Check sheet for the modelled part. Datum: model origin and axes. Units: mm. Face numbers are marked on the shaded views. A direction names the side the tool comes from. Coordinates: 2 decimals unless noted, no trailing zeros. Loops run counter-clockwise (first coordinate to the right, second up) from the corner with the lowest first, then second, coordinate; pieces in that order, holes last. Notation, with made-up numbers: M 27,-2.75 L 41,-2.75 A24 cw 41,15.25 Z; hole C -35,89.5 d1. An arc over 180 degrees is marked long. Write each question's results on one line, items separated by ' | '. Start each with the question number.
Autodesk Inventor part; units mm, degrees
ref_plane "Work Plane1" through (-69.6848, 0, 13.4826) normal (-0.0507, 0, 0.9987) x (0.9987, 0, 0.0507)
ref_plane "YZ Plane" through (0, 0, 0) normal (1, 0, 0) x (0, 1, 0)
ref_plane "XZ Plane" through (0, 0, 0) normal (0, 1, 0) x (-1, 0, 0)
sketch "Sketch1" plane through (0, 0, 0) normal (0, 1, 0) x (-1, 0, 0)
  circle A0 centre (0, 0) radius 19.5
  line L0 (0, 0) -> (69, 0) construction
  circle A1 centre (69, 0) radius 16
  line L1 (69.8116, -15.9794) -> (0.9891, -19.4749)
  line L2 (69.8116, 15.9794) -> (0.9891, 19.4749)
  point P0 (0.9891, 19.4749)
  dimension "d0" = 39
  dimension "d1" = 32
  dimension "d2" = 69
extrude "Extrusion1" add sketch "Sketch1" along normal blind 2.5 contours A0 L2 A1 L1 | A1
sketch "Sketch3" plane through (0, 0, 0) normal (0, 0, 1) x (1, 0, 0)
  line L0 (0, 0) -> (0, 29.1077)
  line L1 (0, 22) -> (-16.5, 22)
  line L2 (-16.5, 22) -> (-16.5, 44)
  line L3 (-16.5, 44) -> (-19.5, 44)
  line L4 (-19.5, 44) -> (-19.5, 2.5)
  line L5 (-19.5, 2.5) -> (-0.9891, 2.5)
  line L6 (-19.5, 2.5) -> (-19.5, 0)
  line L7 (-19.5, 0) -> (-16.5, 0)
  line L8 (-19.5, 0) -> (-0.9891, 0)
  line L9 (-16.5, 0) -> (-16.5, 18)
  line L10 (-16.5, 18) -> (0, 18)
  line L11 (-18, 44) -> (-18, 42)
  line L12 (-18, 42) -> (-19.5, 42)
  line L13 (-4, 18) -> (-4, 19)
  line L14 (-4, 19) -> (-11, 19)
  line L15 (-11, 19) -> (-11, 22)
  point P0 (-16.5, 2.5)
  dimension "d5" = 44
  dimension "d6" = 2
  dimension "d7" = 18
  dimension "d8" = 16.5
  dimension "d10" = 4
  dimension "d11" = 3
  dimension "d12" = 22
  dimension "d13" = 11
  dimension "d14" = 1
revolve "Revolution1" add sketch "Sketch3" angle 360 about axis through (0, 0, 0) along (0, 1, 0) contours L10 L9 L5 L4 L12 L11 L3 L2 L1 L15 L14 L13 | L9 L7 L6 L5
sketch "Sketch4" plane through (0, 2.5, 0) normal (0, 1, 0) x (1, 0, 0)
  line L0 (0, 0) -> (-85, 0)
  arc A0 (-69.8116, 15.9794) -> (-69.8116, -15.9794) centre (-69, 0) ccw
  circle A1 centre (-46.5, 0) radius 7
  circle A2 centre (-69, 0) radius 7
  dimension "d17" = 46.5
  dimension "d18" = 22.5
  dimension "d19" = 14
extrude "Extrusion2" add sketch "Sketch4" along normal blind 2.5
ref_plane "Work Plane1" through (-69.6848, 0, 13.4826) normal (-0.0507, 0, 0.9987) x (0.9987, 0, 0.0507)
sketch "Sketch6" plane through (-69.6848, 0, 13.4826) normal (-0.0507, 0, 0.9987) x (0.9987, 0, 0.0507)
  line L0 (68.9112, 0) -> (68.9112, 13.5)
  line L1 (68.9112, 13.5) -> (49.4112, 13.5)
  line L2 (49.4112, 13.5) -> (29.471, 5)
  line L3 (29.471, 5) -> (7, 5)
  line L4 (7, 5) -> (0, 2.5)
  line L5 (66.9355, 2.5) -> (-1.6211, 2.5)
  line L6 (29.471, 2.5) -> (29.471, 5)
  line L7 (7, 2.5) -> (7, 5)
  line L8 (49.4112, 2.5) -> (49.4112, 42)
  line L9 (7, 5) -> (-7, 5)
  line L10 (0, 5) -> (0, 18.3194) construction
  line L11 (66.9355, 0) -> (-1.6211, 0)
  line L12 (66.9355, 2.5) -> (68.9112, 2.5)
  dimension "d23" = 13.5
  dimension "d24" = 5
extrude "Extrusion3" add sketch "Sketch6" along normal blind 2.5
mirror "Mirror1" about plane through (0, 0, 0) normal (0, 0, 1) of "Extrusion3"
sketch "Sketch7" plane through (0, 0, 0) normal (0, 0, 1) x (1, 0, 0)
  line L0 (-17.1617, 6.6953) -> (-62, 2.52)
  line L1 (-62, 2.5) -> (-62, 5)
  line L2 (-62, 2.52) -> (-62, 2.5)
  line L3 (-10.4025, 2.5) -> (-69.6848, 2.5)
  line L4 (-17.1617, 2.5) -> (-62, 2.5)
  line L5 (-17.1617, 2.5) -> (-17.1617, 6.6953)
  line L6 (-0.9891, 0) -> (-69.8116, 0)
  line L7 (-62, 2.52) -> (-62.2148, 2.5)
  point P0 (0, 0)
  dimension "d27" = 5.32
  dimension "d28" = 2.52
extrude "Extrusion4" add sketch "Sketch7" along normal mid plane 3.5
sketch "Sketch8" plane through (-46.5, 5, 0) normal (0, 1, 0) x (1, 0, 0)
  arc A0 (-6.7777, -1.75) -> (6.7777, -1.75) centre (0, 0) ccw
  circle A1 centre (0, 0) radius 3
  arc A2 (-15.7148, 1.7207) -> (-15.7148, -1.7207) centre (-22.5, 0) ccw
  circle A3 centre (-22.5, 0) radius 3
  point P0 (46.5, 0)
  point P1 (-15.5, 0)
  dimension "d31" = 6
extrude "Extrusion5" cut sketch "Sketch8" against normal through all
sketch "Sketch9" plane through (0, 44, 0) normal (0, 1, 0) x (1, 0, 0)
  circle A0 centre (0, -16) radius 4.5
  line L0 (0, 0) -> (24.199, 0) construction
  circle A1 centre (0, 0) radius 16.5
  circle A2 centre (0, 16) radius 4.5
  point P0 (-4.4983, 15.875)
  point P1 (4.4983, 15.875)
  point P2 (-4.4983, -15.875)
  point P3 (4.4983, -15.875)
  dimension "d34" = 9
  dimension "d35" = 16
extrude "Extrusion6" add sketch "Sketch9" against normal up to surface (22 mm away) contours A1 A0 | A1 A2 picked at (-0.1776, -14.7973) picked at (-0.1776, 14.7973)
sketch "Sketch10" plane through (0, 44, 0) normal (0, 1, 0) x (1, 0, 0)
  arc A0 (4.4983, -15.875) -> (-4.4983, -15.875) centre (0, -16) ccw
  circle A1 centre (0, -16) radius 1.5
  line L0 (0, 0) -> (9.3395, 0) construction
  circle A2 centre (0, 16) radius 1.5
  dimension "d38" = 3
extrude "Extrusion7" cut sketch "Sketch10" against normal blind 4
sketch "Sketch11" plane through (0, 0, 0) normal (0, -1, 0) x (1, 0, 0)
  circle A0 centre (0, 16) radius 1.5
  circle A1 centre (0, 16) radius 2.5
  line L0 (0, 0) -> (10.318, 0)
  circle A2 centre (0, -16) radius 2.5
  dimension "d41" = 5
extrude "Extrusion8" cut sketch "Sketch11" against normal up to surface (40 mm away) contours A0 | A1 | A2
sketch "Sketch12" plane through (0, 44, 0) normal (0, 1, 0) x (1, 0, 0)
  line L0 (36.079, 0) -> (-96.4154, 0)
  line L1 (-96.4154, 0) -> (-96.4154, 28.1723)
  line L2 (-96.4154, 28.1723) -> (36.079, 28.1723)
  line L3 (36.079, 28.1723) -> (36.079, 0)
  point P0 (0, 0)
properties part number "pt1" material "Stainless Steel"
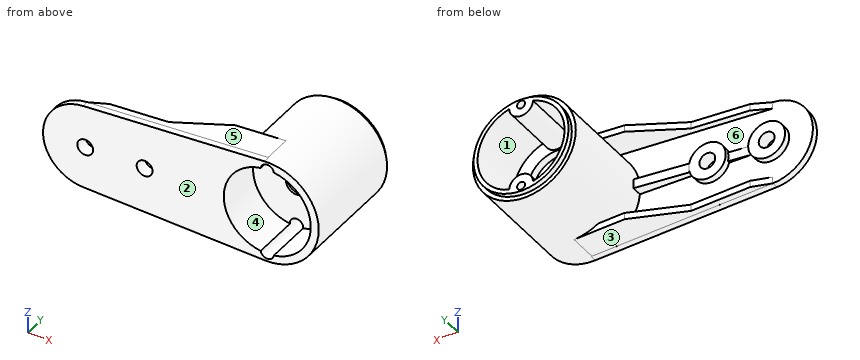
Item 1: Depth check by flat-ended pin: P1, Ø3, axis at x = -72.5, z = -15, coming from the +Y side; P2, Ø2.5, axis at x = 0, z = -16, coming from the -Y side; P3, Ø2, axis at y = 27, z = 10, coming from the -X side; P4, Ø6, axis at y = 28.5, z = 5.5, coming from the +X side. Enter the tip coordinate at first touch or a pass-through.
Item 2: Section check B-B (y = 14.5). Record the cut outline in (x, z).
Item 3: Release check for a two-part mould opening along X. For the marked faces 1, 2 and 3 record: +X half, -X half, draft (parallel to the pull), parting line (faces both ways), or undercut.
Item 4: Section check C-C (x = 0). State how many separate pieces and enclosed holes the cut face has, plus the area to 3 significant figures.
Item 5: Thickness scan on line 1 (Z direction, x = 0, y = 20); line 2 (Z direction, x = 0, y = 41.6); line 3 (Z direction, x = -69, y = 3). Record the ranges inside material, lowest first.
Item 6: Tool access check on the marked faces 4, 5 and 6. Record the directions out of +Z, -Z, +X, -X, +Y, -Y that give a thin tool (end or side, any length) a straight path to the whole face; none if there is none.
Item 7: Section check A-A (y = 33.5). Record the cut outline in (x, z) (3 decimals), plus the area to 3 significant figures.
Computed values:
1) P1: stops at y = 2.5 | P2: passes through | P3: stops at x = -17.3 | P4: stops at x = 19.34
2) outline: C 0,0 d39; hole M -2.48,-16.31 A2.5 ccw 2.48,-16.31 A16.5 ccw 2.48,16.31 A2.5 ccw -2.48,16.31 A16.5 ccw Z
3) face 1: undercut | face 2: draft | face 3: -X half
4) separate pieces: 4 | enclosed holes: 0 | area: 220 mm²
5) line 1: z = -19.5 to -18.5, -13.5 to -11, 11 to 13.5, 18.5 to 19.5 | line 2: z = -19.5 to -17.5, -14.5 to -11.5, 11.5 to 14.5, 17.5 to 19.5 | line 3: z = -7 to -3, 3 to 7
6) face 4: -Y | face 5: +Z, -X, +Y, -Y | face 6: +Y
7) outline: C 0,0 d39; hole M -4.498,-15.875 A4.5 cw 4.498,-15.875 A16.5 ccw 4.498,15.875 A4.5 cw -4.498,15.875 A16.5 ccw Z; hole C 0,-16 d5; hole C 0,16 d5 | area: 369 mm²
